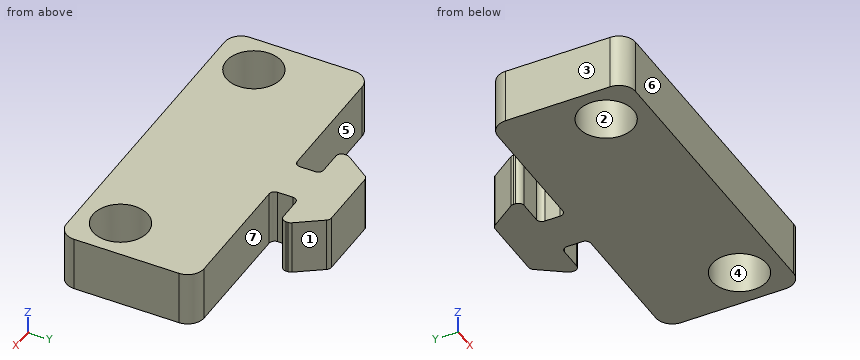
```python
from build123d import *

# Parameters (mm, degrees)
BOSS_EXTRUDE1_DEPTH = 10
BOSS_EXTRUDE2_DEPTH = 10
SKETCH5_R           = 5
CUT_EXTRUDE1_DEPTH  = 44.45158225
FILLET1_R           = 1
FILLET2_R           = 1
FILLET3_R           = 3


with BuildPart() as part:
    # Sketch2 → Boss-Extrude1 (new body)
    with BuildSketch(Plane.XY):
        Polygon((-10, 0), (0, 0), (0, 7), (-6.25480432, 7), (-10, 1.709943763), align=None)
        Polygon((0, 0), (10, 0), (10, 1.709943763), (6.25480432, 7), (0, 7), align=None)
    extrude(amount=BOSS_EXTRUDE1_DEPTH)

    # Sketch4 → Boss-Extrude2 (add)
    with BuildSketch(Plane.XY):
        Polygon((0, 0), (-3.8, 0), (-3.8, -4.8), (-30, -4.8), (-30, -22.686959784), (-30, -23.48), (-30, -29.8), (0, -29.8), align=None)
        Polygon((3.8, 0), (0, 0), (0, -29.8), (30, -29.8), (30, -23.48), (30, -22.686959784), (30, -4.8), (3.8, -4.8), align=None)
    extrude(amount=BOSS_EXTRUDE2_DEPTH)

    # Sketch5 → Cut-Extrude1 (cut, through all)
    with BuildSketch(Plane.XY):
        with Locations((-22.790976064, -22.227391232)):
            Circle(SKETCH5_R)
        with Locations(Location((22.790976064, -22.227391232, 0), (0, 0, 180))):
            Circle(SKETCH5_R)
    extrude(amount=CUT_EXTRUDE1_DEPTH, mode=Mode.SUBTRACT)

    # Fillet1
    fillet1_edges = [part.edges().sort_by_distance(p)[0] for p in [
        (-10, 0, 5),
        (-10, 1.709943763, 5),
        (-6.25480432, 7, 5),
        (6.25480432, 7, 5),
        (10, 1.709943763, 5),
        (10, 0, 5),
    ]]
    fillet(fillet1_edges, radius=FILLET1_R)

    # Fillet2
    fillet2_edges = [part.edges().sort_by_distance(p)[0] for p in [
        (3.8, -4.8, 5),
        (3.8, 0, 5),
        (-3.8, 0, 5),
        (-3.8, -4.8, 5),
    ]]
    fillet(fillet2_edges, radius=FILLET2_R)

    # Fillet3
    fillet3_edges = [part.edges().sort_by_distance(p)[0] for p in [
        (-30, -29.8, 5),
        (30, -29.8, 5),
        (30, -4.8, 5),
        (-30, -4.8, 5),
    ]]
    fillet(fillet3_edges, radius=FILLET3_R)


solid = part.part
```
Geometry check sheet. Reference: the model listing, model coordinates, mm. Face numbers are marked on the shaded views. A direction names the side the tool comes from. Round coordinates to 2 decimals unless told otherwise and drop trailing zeros. Loops run counter-clockwise (first coordinate to the right, second up) from the corner with the lowest first, then second, coordinate; pieces in that order, holes last. Notation, with made-up numbers: (41, 32) - (76, 32) arc R27 cw to (76, 52) - close; hole circle Ø5 at (71.25, 51.5). An arc over 180 degrees is marked (long way). Use a Markdown table: item, result.
Q1. Cross-section at B-B on z = 2.5. State how many separate pieces and enclosed holes the cut face has, plus the area to 3 significant figures.
Solutions:
| item | result |
|---|---|
| separate pieces | 1 |
| enclosed holes | 2 |
| area | 1,490 mm2 |
Q2. Access from +Z, -Z, +X, -X, +Y, -Y to the whole of each face (thin tool, end or side, straight path). Record for the marked faces 5, 6 and 7.
Solutions:
| item | result |
|---|---|
| face 5 | +Z, -Z, -X |
| face 6 | +Z, -Z, +X, -X, -Y |
| face 7 | +Z, -Z, +X |
Q3. Material ranges on line 1 (Y direction, x = 5, z = 3.5); line 2 (X direction, y = -25.5, z = 7.25); line 3 (X direction, y = -25, z = 6.75), recorded low to high.
Solutions:
| item | result |
|---|---|
| line 1 | y = -29.8 to -4.8, 0 to 7 |
| line 2 | x = -30 to -26.57, -19.01 to 19.01, 26.57 to 30 |
| line 3 | x = -30 to -26.95, -18.63 to 18.63, 26.95 to 30 |
Q4. Cross-section at A-A on x = 24.5. Record the cut outline in (y, z), plus the area to 3 significant figures.
Solutions:
| item | result |
|---|---|
| outline | (-29.8, 0) - (-26.93, 0) - (-26.93, 10) - (-29.8, 10) - close; (-17.53, 0) - (-4.8, 0) - (-4.8, 10) - (-17.53, 10) - close |
| area | 156 mm2 |
Q5. Cross-section at D-D on x = 13.5. Record the cut outline in (y, z), plus the area to 3 significant figures.
Solutions:
| item | result |
|---|---|
| outline | (-29.8, 0) - (-4.8, 0) - (-4.8, 10) - (-29.8, 10) - close |
| area | 250 mm2 |
Q6. Draft check along X on the marked faces 1, 2, 3 and 4. Enter one of: released by +X, released by -X, zero draft, split by the parting line, or undercut.
Solutions:
| item | result |
|---|---|
| face 1 | released by +X |
| face 2 | undercut |
| face 3 | released by -X |
| face 4 | undercut |
Q7. Cross-section at C-C on y = -26. Record the cut outline in (x, z).
Solutions:
| item | result |
|---|---|
| outline | (-30, 0) - (-26.07, 0) - (-26.07, 10) - (-30, 10) - close; (-19.51, 0) - (19.51, 0) - (19.51, 10) - (-19.51, 10) - close; (26.07, 0) - (30, 0) - (30, 10) - (26.07, 10) - close |
Q8. Go/stop test with flat-tipped pins: P1, Ø3, axis at x = 16.5, z = 7, coming from the +Y side; P2, Ø1.4, axis at y = -3, z = 4.5, coming from the +X side; P3, Ø0.8, axis at y = -2, z = 3, coming from the -X side; P4, Ø8, axis at x = -22.79, y = -22.23, coming from the -Z side. Record where each tip stops, or that it passes through.
Solutions:
| item | result |
|---|---|
| P1 | stops at y = -4.8 |
| P2 | stops at x = 3.8 |
| P3 | stops at x = -3.8 |
| P4 | passes through |
